from build123d import *

# Parameters (mm, degrees)
F1_W     = 76.2
F1_H     = 76.2
F2_DEPTH = 76.2
F3_R     = 12.7
F4_DEPTH = 76.201


with BuildPart() as f2:
    # F1 (on face) → F2 (new body)
    with BuildSketch(Plane.XY):
        Rectangle(F1_W, F1_H)
    extrude(amount=F2_DEPTH)

    # F3 (on face) → F4 (cut, through all)
    with BuildSketch(Plane.XY.offset(76.2)):
        Circle(F3_R)
    extrude(amount=-F4_DEPTH, mode=Mode.SUBTRACT)


solid = f2.part
Geometry: final body of the model. Coordinates: model frame, mm. Coordinates: 2 decimals unless noted, no trailing zeros. Loops run counter-clockwise (first coordinate to the right, second up) from the corner with the lowest first, then second, coordinate; pieces in that order, holes last. Notation, with made-up numbers: M -14.5,-25 L 29.5,-25 A5 ccw 29.5,-18 Z; hole C -7,-15.5 d1. An arc over 180 degrees is marked long. One line per item, written item: value. Start each with the question number.
1) Cut plane A-A (y = 0). Return loops of the section in (x, z), then the cut area to 3 significant figures.
2) Cut plane C-C (z = 14.5). Return loops of the section in (x, y).
3) Material intervals for L1, parallel to Y at x = 0, z = 39.5; L2, parallel to X at y = 3.5, z = 35; L3, parallel to X at y = 3, z = 59.5, sorted ascending. Write a range as from..to.
4) Cut plane B-B (x = -7.5). Return loops of the section in (y, z), then the cut area to 3 significant figures.
5) Draft query along X for faces 1 (the cylindrical face through (-2.75, -12.4, 38.63)), 2 (the flat face through (-1, -38.1, 38)), 3 (the flat face through (38.1, -1, 38)). Return one class per face: released by +X, released by -X, zero draft, split by the parting line, or undercut.
6) Pin query (flat end, axial travel): P1, Ø23, axis at x = 0, y = 0, coming from the -Z side. Return the tip coordinate at first contact, or that it passes through.
Evaluation:
1. outline: M -38.1,0 L -12.7,0 L -12.7,76.2 L -38.1,76.2 Z; M 12.7,0 L 38.1,0 L 38.1,76.2 L 12.7,76.2 Z
1. area: 3,870 mm^2
2. outline: M -38.1,-38.1 L 38.1,-38.1 L 38.1,38.1 L -38.1,38.1 Z; hole C 0,0 d25.4
3. L1: -38.1..-12.7, 12.7..38.1
3. L2: -38.1..-12.21, 12.21..38.1
3. L3: -38.1..-12.34, 12.34..38.1
4. outline: M -38.1,0 L -10.25,0 L -10.25,76.2 L -38.1,76.2 Z; M 10.25,0 L 38.1,0 L 38.1,76.2 L 10.25,76.2 Z
4. area: 4,240 mm^2
5. face 1: undercut
5. face 2: zero draft
5. face 3: released by +X
6. P1: through
